The listing builds one solid part. Answer for the finished solid, in the listing's coordinates (mm). Face numbers are marked on the shaded views. Round coordinates to 2 decimals unless told otherwise and drop trailing zeros. Write each loop counter-clockwise with the first axis right and the second up, starting at its lowest first coordinate (ties: lowest second). Pieces come first, ordered by that corner, then holes. Notation, with made-up numbers: (-9.75, 71.25) -> (16.25, 71.25) arc R17 ccw to (16.25, 98.25) -> close; hole circle Ø9 at (21, -24.5). An arc over 180 degrees is marked (long way). Write each question's results on one line, items separated by ' | '. Start each with the question number.
```python
from build123d import *

# Parameters (mm, degrees)
F0_W     = 127
F0_H     = 127
F1_DEPTH = 25.4
F2_R     = 31.75
F3_DEPTH = 25.401
F5_DEPTH = 127.001


with BuildPart() as f1:
    # F0 (on Front) → F1 (new body)
    with BuildSketch(Plane.XZ):
        with Locations((63.5, 63.5)):
            Rectangle(F0_W, F0_H)
    extrude(amount=F1_DEPTH)

    # F2 (on face) → F3 (cut, through all)
    with BuildSketch(Plane.XZ.offset(25.4)):
        with Locations((63.5, 63.5)):
            Circle(F2_R)
    extrude(amount=-F3_DEPTH, mode=Mode.SUBTRACT)

    # F4 (on face) → F5 (cut, through all)
    with BuildSketch(Plane.XY.offset(127)):
        Polygon((111.601122, -5.075065), (103.562877, -9.875687), (106.577218, -18.918719), (116.17846, -20.593353), (118.857875, -11.661964), align=None)
    extrude(amount=-F5_DEPTH, mode=Mode.SUBTRACT)


solid = f1.part
```
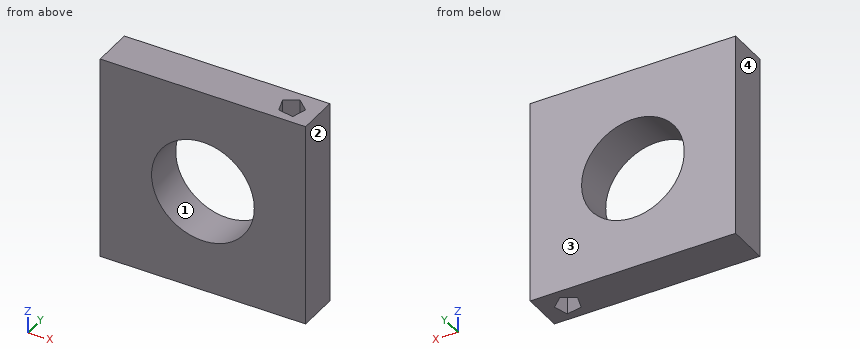
Q1. The part is cut by section B-B, the plane y = -14.75. Write down the section's boundary in (x, z), then the cut area to 3 significant figures.
Q2. Find the intervals of material crossed by line 1 (X direction, y = -11, z = 62); line 2 (X direction, y = -12, z = 53.5); line 3 (X direction, y = -14.5, z = 96.5), in increasing order.
Q3. The part is cut by section D-D, the plane y = -2.75. Write down the section's boundary in (x, z).
Q4. Determine the mould class of the marked faces 1, 2, 3 and 4 for opening direction X: pulls with the +X half, pulls with the -X half, needs draft (parallel to the pull), parting line crosses it, or undercut.
Q5. The part is cut by section A-A, the plane z = 63.5. Write down the section's boundary in (x, y), then the cut area to 3 significant figures.
Q6. The part is cut by section C-C, the plane x = 69. Write down the section's boundary in (y, z), then the cut area to 3 significant figures.
Answers follow:
1) outline: (0, 0) -> (105.19, 0) -> (105.19, 127) -> (0, 127) -> close; (117.93, 0) -> (127, 0) -> (127, 127) -> (117.93, 127) -> close; hole circle Ø63.5 at (63.5, 63.5) | area: 11,300 mm^2
2) line 1: 0 to 31.79, 95.21 to 103.94, 118.13 to 127 | line 2: 0 to 33.37, 93.63 to 104.27, 118.76 to 127 | line 3: 0 to 105.1, 118.01 to 127
3) outline: (0, 0) -> (127, 0) -> (127, 127) -> (0, 127) -> close; hole circle Ø63.5 at (63.5, 63.5)
4) face 1: undercut | face 2: pulls with the +X half | face 3: needs draft | face 4: pulls with the -X half
5) outline: (0, -25.4) -> (31.75, -25.4) -> (31.75, 0) -> (0, 0) -> close; (95.25, -25.4) -> (127, -25.4) -> (127, 0) -> (95.25, 0) -> close; hole (103.56, -9.88) -> (106.58, -18.92) -> (116.18, -20.59) -> (118.86, -11.66) -> (111.6, -5.08) -> close | area: 1,460 mm^2
6) outline: (-25.4, 0) -> (0, 0) -> (0, 32.23) -> (-25.4, 32.23) -> close; (-25.4, 94.77) -> (0, 94.77) -> (0, 127) -> (-25.4, 127) -> close | area: 1,640 mm^2
